from build123d import *

# Parameters (mm, degrees)
BOSS_EXTRUDE1_DEPTH = 2.5
SKETCH2_W           = 5.2
SKETCH2_H           = 5.2
BOSS_EXTRUDE2_DEPTH = 4
FILLET1_R           = 1
SKETCH3_R           = 2.1
CUT_EXTRUDE1_DEPTH  = 23.707487752


with BuildPart() as part:
    # Sketch1 → Boss-Extrude1 (new body)
    with BuildSketch(Plane(origin=(0, 0, 0), x_dir=(0, 1, 0), z_dir=(0, 0, 1))):
        with BuildLine():
            Line((0, 6.7), (14, 6.7))
            ThreePointArc((14, 6.7), (20.7, 0), (14, -6.7))
            Line((14, -6.7), (0, -6.7))
            ThreePointArc((0, -6.7), (-6.7, 0), (0, 6.7))
        make_face()
    extrude(amount=BOSS_EXTRUDE1_DEPTH)

    # Sketch2 → Boss-Extrude2 (add)
    with BuildSketch(Plane.XY.offset(2.5)):
        with Locations((0, -2.6)):
            Rectangle(SKETCH2_W, SKETCH2_H)
        with Locations((0, 16.6)):
            Rectangle(SKETCH2_W, SKETCH2_H)
    extrude(amount=BOSS_EXTRUDE2_DEPTH)

    # Fillet1
    fillet1_edges = [part.edges().sort_by_distance(p)[0] for p in [
        (-2.6, 0, 4.5),
        (-2.6, -5.2, 4.5),
        (2.6, -5.2, 4.5),
        (2.6, 0, 4.5),
        (-2.6, -2.6, 6.5),
        (0, -5.2, 6.5),
        (2.6, -2.6, 6.5),
        (0, 0, 6.5),
        (-2.6, 14, 4.5),
        (2.6, 14, 4.5),
        (2.6, 19.2, 4.5),
        (-2.6, 19.2, 4.5),
        (0, 14, 6.5),
        (2.6, 16.6, 6.5),
        (0, 19.2, 6.5),
        (-2.6, 16.6, 6.5),
    ]]
    fillet(fillet1_edges, radius=FILLET1_R)

    # Sketch3 → Cut-Extrude1 (cut, through all)
    with BuildSketch(Plane.XY.offset(6.5)):
        with Locations((0, 16.6)):
            Circle(SKETCH3_R)
        with Locations(Location((0, -2.6, 0), (0, 0, 319.632406456))):
            Circle(SKETCH3_R)
    extrude(amount=-CUT_EXTRUDE1_DEPTH, mode=Mode.SUBTRACT)


solid = part.part
Here's how the part is built. I have some questions about the finished solid (model axes, mm). A direction names the side the tool comes from. Coordinates: 2 decimals unless noted, no trailing zeros. Order: outer loops, then holes, each group sorted by start corner. A loop starts at its lowest first (then second) coordinate and runs counter-clockwise, first axis right, second up. Notation, with made-up numbers: (-30, 7.5) -> (28, 7.5) arc R6 cw to (28, 15.5) -> close; hole circle Ø3 at (-38.5, 70.5). An arc over 180 degrees is marked (long way). Answer in a Markdown table with one row per item.
(1) Thinking about a two-plate mould opening in X: for faces 4 (the face through (0, 19.2, 4)), 5 (the face through (2.4, 16.6, 6.1)), 6 (the face through (0.957, -4.469, 3.296)), 7 (the face through (1.13, 18.37, 3.3)), which applies, +X half, -X half, draft (parallel to the pull), parting line (faces both ways), or undercut?
Answer key:
| item | result |
|---|---|
| face 4 | draft |
| face 5 | +X half |
| face 6 | undercut |
| face 7 | undercut |
(2) I want a section at D-D on y = -2. List the corners of the cut face in (x, z) for me, then the cut area to 3 significant figures.
Answer key:
| item | result |
|---|---|
| outline | (-6.39, 0) -> (-2.01, 0) -> (-2.01, 6.41) arc R1 ccw to (-2.6, 5.5) -> (-2.6, 2.5) -> (-6.39, 2.5) -> close; (2.01, 0) -> (6.39, 0) -> (6.39, 2.5) -> (2.6, 2.5) -> (2.6, 5.5) arc R1 ccw to (2.01, 6.41) -> close |
| area | 26.2 mm^2 |
(3) I want a section at B-B on x = 0. List the corners of the cut face in (y, z) for me.
Answer key:
| item | result |
|---|---|
| outline | (-6.7, 0) -> (-4.7, 0) -> (-4.7, 6.37) arc R1 ccw to (-5.2, 5.5) -> (-5.2, 2.5) -> (-6.7, 2.5) -> close; (-0.5, 0) -> (14.5, 0) -> (14.5, 6.37) arc R1 ccw to (14, 5.5) -> (14, 2.5) -> (0, 2.5) -> (0, 5.5) arc R1 ccw to (-0.5, 6.37) -> close; (18.7, 0) -> (20.7, 0) -> (20.7, 2.5) -> (19.2, 2.5) -> (19.2, 5.5) arc R1 ccw to (18.7, 6.37) -> close |
(4) Please list where these lines run through material, in increasing order: probe 1 along Y at (x, z) = (0, 3.5); probe 2 along Y at (x, z) = (0, 1.25); probe 3 along Y at (x, z) = (-0.5, 4).
Answer key:
| item | result |
|---|---|
| probe 1 | -5.2 to -4.7, -0.5 to 0, 14 to 14.5, 18.7 to 19.2 |
| probe 2 | -6.7 to -4.7, -0.5 to 14.5, 18.7 to 20.7 |
| probe 3 | -5.2 to -4.64, -0.56 to 0, 14 to 14.56, 18.64 to 19.2 |
(5) On a 3-axis mill with a long thin cutter (end or side, diameter ignored), from which of +Z, -Z, +X, -X, +Y, -Y can I reach the whole of each face in a straight line? I mean faces 1 (the face through (2.299, 18.915, 4.021)), 2 (the face through (2.6, -3, 4)), 3 (the face through (0, 14.2, 6.1)). Say none if no direction works.
Answer key:
| item | result |
|---|---|
| face 1 | +Z, +X, +Y |
| face 2 | +Z, +X, +Y, -Y |
| face 3 | +Z, +X, -X |
(6) I want a section at A-A on z = 5.25. List the corners of the cut face in (x, y) for me, then the cut area to 3 significant figures.
Answer key:
| item | result |
|---|---|
| outline | (-2.6, -4.2) arc R1 ccw to (-1.6, -5.2) -> (1.6, -5.2) arc R1 ccw to (2.6, -4.2) -> (2.6, -1) arc R1 ccw to (1.6, 0) -> (-1.6, 0) arc R1 ccw to (-2.6, -1) -> close; (-2.6, 15) arc R1 ccw to (-1.6, 14) -> (1.6, 14) arc R1 ccw to (2.6, 15) -> (2.6, 18.2) arc R1 ccw to (1.6, 19.2) -> (-1.6, 19.2) arc R1 ccw to (-2.6, 18.2) -> close; hole circle Ø4.2 at (0, -2.6); hole circle Ø4.2 at (0, 16.6) |
| area | 24.7 mm^2 |
(7) Will these pins go through, and if not, where does the flat tip stop? pin 1 Ø3.5 at (y, z) = (-3.5, 4) entering from -X; pin 2 Ø0.9 at (y, z) = (17, 3.5) entering from +X; pin 3 Ø1.5 at (x, z) = (0, 3.5) entering from +Y.
Answer key:
| item | result |
|---|---|
| pin 1 | x = -6.18 |
| pin 2 | x = 2.6 |
| pin 3 | y = 19.2 |
(8) I want a section at C-C on z = 1.5. List the corners of the cut face in (x, y) for me, then the cut area to 3 significant figures.
Answer key:
| item | result |
|---|---|
| outline | (-6.7, 0) arc R6.7 ccw to (6.7, 0) -> (6.7, 14) arc R6.7 ccw to (-6.7, 14) -> close; hole circle Ø4.2 at (0, -2.6); hole circle Ø4.2 at (0, 16.6) |
| area | 301 mm^2 |
